```python
from build123d import *

# Parameters (mm, degrees)
ESBO_O1_R                = 9.5
RESSALTO_EXTRUS_O1_DEPTH = 11
FILETE1_R                = 5
ESBO_O2_R                = 5.1000000000000005
CORTE_EXTRUS_O1_DEPTH    = 6
FILETE2_R                = 5
FILETE4_R                = 2


with BuildPart() as part:
    # Esboço1 → Ressalto-extrusão1 (new body)
    with BuildSketch(Plane(origin=(0, 0, 0), x_dir=(0, 0, -1), z_dir=(1, 0, 0))):
        Circle(ESBO_O1_R)
        with BuildLine():
            Line((9.500000000000002, -20), (9.5, 0))
            ThreePointArc((9.5, -2.33e-15), (-1.75e-15, -9.5), (-9.5, 1.16e-15))
            Line((-9.5, 0), (-9.5, -30.5))
            ThreePointArc((-9.5, -30.5), (2.298839010018332, -29.40980392289032), (9.5, -20))
        make_face()
    extrude(amount=-RESSALTO_EXTRUS_O1_DEPTH)

    # Filete1
    filete1_edges = [part.edges().sort_by_distance(p)[0] for p in [
        (-5.5, -30.5, 9.5),
    ]]
    fillet(filete1_edges, radius=FILETE1_R)

    # Esboço2 → Corte-extrusão1 (cut)
    with BuildSketch(Plane(origin=(0, 0, 0), x_dir=(0, 0, -1), z_dir=(1, 0, 0))):
        Circle(ESBO_O2_R)
    extrude(amount=-CORTE_EXTRUS_O1_DEPTH, mode=Mode.SUBTRACT)

    # Filete2
    # the kernel refuses this fillet: 5 mm, written as the material it takes off along each edge
    with BuildSketch(Plane(origin=(-11, -16.482034889709183, 4.845454403055449), x_dir=(0, -0.9993747520623889, -0.035356823107268454), z_dir=(0, -0.035356823107268454, 0.9993747520623889))) as filete2_piece_1:
        with BuildLine():
            CenterArc((14.770515920148714 - FILETE2_R, FILETE2_R), FILETE2_R, 270, 90)
            Line((14.770515920148714 - FILETE2_R, 0), (14.770515920148714 - FILETE2_R, -FILETE2_R * 0.02))
            Line((14.770515920148714 - FILETE2_R, -FILETE2_R * 0.02), (14.770515920148714 + FILETE2_R * 0.02, -FILETE2_R * 0.02))
            Line((14.770515920148714 + FILETE2_R * 0.02, -FILETE2_R * 0.02), (14.770515920148714 + FILETE2_R * 0.02, FILETE2_R))
            Line((14.770515920148714 + FILETE2_R * 0.02, FILETE2_R), (14.770515920148714, FILETE2_R))
        make_face()
    revolve(axis=Axis((-11, -16.482034889709183, 4.845454403055449), (1, 0, 0)), revolution_arc=93.59555420647537, mode=Mode.SUBTRACT)
    with BuildSketch(Plane(origin=(-11, -25, -9.500000000000002), x_dir=(1, 0, 0), z_dir=(0, 1, 9e-17))) as filete2_piece_2:
        with BuildLine():
            CenterArc((FILETE2_R, -FILETE2_R), FILETE2_R, 90, 90)
            Line((0, -FILETE2_R), (-FILETE2_R * 0.02, -FILETE2_R))
            Line((-FILETE2_R * 0.02, -FILETE2_R), (-FILETE2_R * 0.02, FILETE2_R * 0.02))
            Line((-FILETE2_R * 0.02, FILETE2_R * 0.02), (FILETE2_R, FILETE2_R * 0.02))
            Line((FILETE2_R, FILETE2_R * 0.02), (FILETE2_R, 0))
        make_face()
    extrude(amount=25, mode=Mode.SUBTRACT)
    with BuildSketch(Plane(origin=(-11, -26.246441814929426, 4.5), x_dir=(0, 0, 1), z_dir=(0, 1, 0))) as filete2_piece_3:
        with BuildLine():
            CenterArc((5 - FILETE2_R, FILETE2_R), FILETE2_R, 270, 90)
            Line((5 - FILETE2_R, 0), (5 - FILETE2_R, -FILETE2_R * 0.02))
            Line((5 - FILETE2_R, -FILETE2_R * 0.02), (5, -FILETE2_R * 0.02))
            Line((5, -FILETE2_R * 0.02), (5 + FILETE2_R * 0.02, 0))
            Line((5 + FILETE2_R * 0.02, 0), (5 + FILETE2_R * 0.02, FILETE2_R))
            Line((5 + FILETE2_R * 0.02, FILETE2_R), (5, FILETE2_R))
        make_face()
    revolve(axis=Axis((-11, -26.246441814929426, 4.5), (1, 0, 0)), revolution_arc=92.02621905507084, mode=Mode.SUBTRACT)
    with BuildSketch(Plane(origin=(-11, 0, 0), x_dir=(0, 0, -1), z_dir=(0, -1, 0))) as filete2_piece_4:
        with BuildLine():
            CenterArc((9.5 - FILETE2_R, FILETE2_R), FILETE2_R, 270, 90)
            Line((9.5 - FILETE2_R, 0), (9.5 - FILETE2_R, -FILETE2_R * 0.02))
            Line((9.5 - FILETE2_R, -FILETE2_R * 0.02), (9.5 + FILETE2_R * 0.02, -FILETE2_R * 0.02))
            Line((9.5 + FILETE2_R * 0.02, -FILETE2_R * 0.02), (9.5 + FILETE2_R * 0.02, FILETE2_R))
            Line((9.5 + FILETE2_R * 0.02, FILETE2_R), (9.5, FILETE2_R))
        make_face()
    revolve(axis=Axis((-11, 0, 0), (1, 0, 0)), revolution_arc=180, mode=Mode.SUBTRACT)
    with BuildSketch(Plane(origin=(-11, 0, 9.5), x_dir=(1, 0, 0), z_dir=(0, -1, 0))) as filete2_piece_5:
        with BuildLine():
            CenterArc((FILETE2_R, -FILETE2_R), FILETE2_R, 90, 90)
            Line((0, -FILETE2_R), (-FILETE2_R * 0.02, -FILETE2_R))
            Line((-FILETE2_R * 0.02, -FILETE2_R), (-FILETE2_R * 0.02, FILETE2_R * 0.02))
            Line((-FILETE2_R * 0.02, FILETE2_R * 0.02), (FILETE2_R, FILETE2_R * 0.02))
            Line((FILETE2_R, FILETE2_R * 0.02), (FILETE2_R, 0))
        make_face()
    extrude(amount=26.246441814929426, mode=Mode.SUBTRACT)

    # Filete4
    # the kernel refuses this fillet: 2 mm, written as the material it takes off along each edge
    with BuildSketch(Plane(origin=(0, -26.246441814929426, 4.5), x_dir=(0, 0, 1), z_dir=(0, 1, 0))) as filete4_piece_1:
        with BuildLine():
            CenterArc((5 - FILETE4_R, -FILETE4_R), FILETE4_R, 6.36e-15, 90)
            Line((5, -FILETE4_R), (5, 0))
            Line((5, 0), (5 - FILETE4_R, 0))
        make_face()
    revolve(axis=Axis((0, -26.246441814929426, 4.5), (1, 0, 0)), revolution_arc=92.02621905507084, mode=Mode.SUBTRACT)
    with BuildSketch(Plane(origin=(0, -25, -9.500000000000002), x_dir=(0, -9e-17, 1), z_dir=(0, 1, 9e-17))) as filete4_piece_2:
        with BuildLine():
            CenterArc((FILETE4_R, -FILETE4_R), FILETE4_R, 90, 90)
            Line((0, -FILETE4_R), (0, 0))
            Line((0, 0), (FILETE4_R, 0))
        make_face()
    extrude(amount=25, mode=Mode.SUBTRACT)
    with BuildSketch(Plane(origin=(0, -16.482034889709183, 4.845454403055449), x_dir=(0, -0.9993747520623889, -0.035356823107268454), z_dir=(0, -0.035356823107268454, 0.9993747520623889))) as filete4_piece_3:
        with BuildLine():
            CenterArc((14.770515920148714 - FILETE4_R, -FILETE4_R), FILETE4_R, 6.36e-15, 90)
            Line((14.770515920148714, -FILETE4_R), (14.770515920148714, 0))
            Line((14.770515920148714, 0), (14.770515920148714 - FILETE4_R, 0))
        make_face()
    revolve(axis=Axis((0, -16.482034889709183, 4.845454403055449), (1, 0, 0)), revolution_arc=93.59555420647538, mode=Mode.SUBTRACT)
    with BuildSketch(Plane(origin=(0, 0, 9.5), x_dir=(0, 0, -1), z_dir=(0, -1, 0))) as filete4_piece_4:
        with BuildLine():
            CenterArc((FILETE4_R, -FILETE4_R), FILETE4_R, 90, 90)
            Line((0, -FILETE4_R), (0, 0))
            Line((0, 0), (FILETE4_R, 0))
        make_face()
    extrude(amount=26.246441814929426, mode=Mode.SUBTRACT)
    with BuildSketch(Plane(origin=(0, 0, 0), x_dir=(0, 0, -1), z_dir=(0, -1, 0))) as filete4_piece_5:
        with BuildLine():
            CenterArc((9.5 - FILETE4_R, -FILETE4_R), FILETE4_R, 6.36e-15, 90)
            Line((9.5, -FILETE4_R), (9.5, 0))
            Line((9.5, 0), (9.5 - FILETE4_R, 0))
        make_face()
    revolve(axis=Axis((0, 0, 0), (1, 0, 0)), revolution_arc=180, mode=Mode.SUBTRACT)


solid = part.part
```
Could you check a few things on this model? Use its own coordinates, in mm. Round coordinates to 2 decimals unless told otherwise and drop trailing zeros. Loops run counter-clockwise (first coordinate to the right, second up) from the corner with the lowest first, then second, coordinate; pieces in that order, holes last. Notation, with made-up numbers: (20, 11.25) -> (56, 11.25) arc R24 cw to (56, 28.25) -> close; hole circle Ø5 at (48, 29). An arc over 180 degrees is marked (long way). Put each result on its own line as item: value.
Q1. I want a section at A-A on x = -4.25. Write out the boundary of the cut face in (y, z).
Checks:
outline: (-31.24, 4.32) arc R14.77 ccw to (-20, -9.5) -> (0, -9.5) arc R9.5 ccw to (0, 9.5) -> (-26.25, 9.5) arc R5 ccw to start; hole circle Ø10.2 at (0, 0)
Q2. Thinking about a two-plate mould opening in Z: for faces 1 (the cylindrical face through (-3.972, 9.498, -0.209)), 2 (the cylindrical face through (-2.958, -1.953, -4.711)), 3 (the flat face through (-6, 0, 0)), 4 (the flat face through (-4, -13, 9.5)), which applies, pulls with the +Z half, pulls with the -Z half, needs draft (parallel to the pull), parting line crosses it, or undercut?
Checks:
face 1: parting line crosses it
face 2: undercut
face 3: undercut
face 4: pulls with the +Z half
Q3. I want a section at C-C on y = -0.5. Write out the boundary of the cut face in (x, z).
Checks:
outline: (-11, -4.5) arc R5 ccw to (-6, -9.5) -> (-2, -9.5) arc R2 ccw to (0, -7.5) -> (0, -5.08) -> (-6, -5.08) -> (-6, 5.08) -> (0, 5.08) -> (0, 7.5) arc R2 ccw to (-2, 9.5) -> (-6, 9.5) arc R5 ccw to (-11, 4.5) -> close
Q4. For pin 1 Ø3 at (y, z) = (0.5, -1.5) entering from +X; pin 2 Ø1 at (x, y) = (-7.5, -16.5) entering from -Z; pin 3 Ø5 at (x, z) = (-9, -1) entering from +Y; pin 4 Ø1 at (y, z) = (-21.5, -1) entering from +X, each with a flat end and sliding along its axis, tell me the tip position at first contact or that it passes through.
Checks:
pin 1: x = -6
pin 2: z = -9.4
pin 3: y = 9.46
pin 4: x = 0
Q5. Please list where these lines run through material, in increasing order: line 1 (X direction, y = -0.5, z = -1); line 2 (Y direction, x = -2.95, z = 0); line 3 (Z direction, x = -10, y = -14). Write a range as from..to.
Checks:
line 1: -11..-6
line 2: -30.44..-5.1, 5.1..9.5
line 3: -7.5..7.5
Q6. I want a section at B-B on y = -11.5. Write out the boundary of the cut face in (x, z), and give its area (3 significant figures).
Checks:
outline: (-11, -4.5) arc R5 ccw to (-6, -9.5) -> (-2, -9.5) arc R2 ccw to (0, -7.5) -> (0, 7.5) arc R2 ccw to (-2, 9.5) -> (-6, 9.5) arc R5 ccw to (-11, 4.5) -> close
area: 197 mm2
